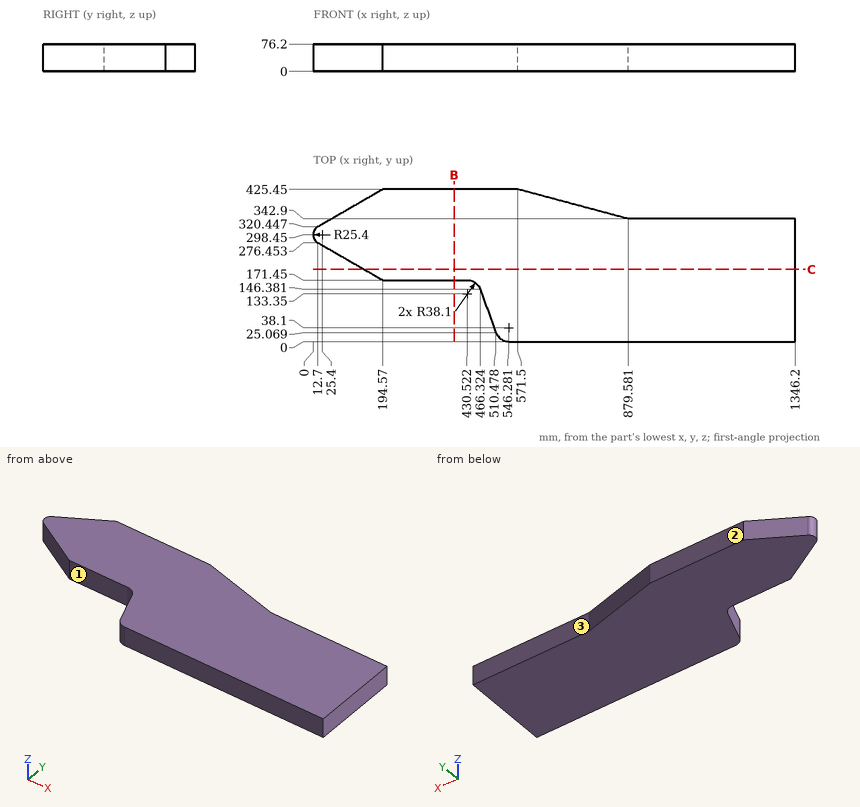
The drawing under review shows one solid part. Ordinate dimensions are in mm from its lowest x, y, z. A direction names the side the tool comes from. Round coordinates to 2 decimals unless told otherwise and drop trailing zeros. Loops run counter-clockwise (first coordinate to the right, second up) from the corner with the lowest first, then second, coordinate; pieces in that order, holes last. Notation, with made-up numbers: (45.5, 16) - (84.5, 16) arc R20 ccw to (84.5, 40) - close; hole circle Ø2 at (29, 62). An arc over 180 degrees is marked (long way). Use one line per item in the form item = value.
Item 1: Consider section B-B on x = 393.5. Write out the cut boundary in (y, z).
Answers:
outline = (171.45, 0) - (425.45, 0) - (425.45, 76.2) - (171.45, 76.2) - close
Item 2: For line 1 (Y direction, x = 1174.5, z = 28.5); line 2 (X direction, y = 25.5, z = 16); line 3 (Y direction, x = 767, z = 64.5) (1 decimal), list the stretches that pass through material, from the lowest coordinate up.
Answers:
line_1 = 0 to 342.9
line_2 = 510.32 to 1346.2
line_3 = 0 to 373.1
Item 3: Tool access review of the marked faces 1, 2 and 3: name each direction out of +Z, -Z, +X, -X, +Y, -Y from which nothing blocks a thin tool from reaching the whole face with its end or side.
Answers:
face_1 = +Z, -Z, -X, -Y
face_2 = +Z, -Z, +X, -X, +Y
face_3 = +Z, -Z, +X, +Y
Item 4: Consider section C-C on y = 201.5. Write out the cut boundary in (x, z).
Answers:
outline = (142.52, 0) - (1346.2, 0) - (1346.2, 76.2) - (142.52, 76.2) - close
Item 5: Clearance check with flat-ended pins moving along their axes: P1, Ø3, axis at y = 178, z = 16.5, coming from the -X side (1 decimal); P2, Ø6, axis at y = 340.5, z = 46, coming from the -X side (1 decimal). State where each tip first meets the part, or that it passes through.
Answers:
P1 = 180.6
P2 = 42.2
